Could you check a few things on this model? Use its own coordinates, in mm. A direction names the side the tool comes from. Give positions to 0.01 mm unless a question says otherwise; leave off trailing zeros. Write each loop counter-clockwise with the first axis right and the second up, starting at its lowest first coordinate (ties: lowest second). Pieces come first, ordered by that corner, then holes. Notation, with made-up numbers: M 56,36.25 L 109,36.25 A16 ccw 109,58.25 Z; hole C 11,57.25 d1. An arc over 180 degrees is marked long. Use one line per item in the form item = value.
from build123d import *

# Parameters (mm, degrees)
F0_W          = 250
F0_H          = 52
F1_DEPTH      = 19.2
F2_SIZE2      = 2.017991
F2_SIZE       = 19.19999
F3_SIZE2      = 2.017991
F3_SIZE       = 19.19999
F4_R          = 6.5
F5_DEPTH      = 1.7951503396
F7_DEPTH      = 58.4841370583
F7_DEPTH_BACK = 301.5629071742
F8_R          = 0.55
F9_DEPTH      = 0.5
F10_R         = 0.49999
F11_R         = 0.49999
F12_R         = 13.25
F13_DEPTH     = 4
F14_W         = 21
F14_H         = 8
F14_H_2       = 8.9314985695
F15_DEPTH     = 4


# Not quite as in the source:
# - a fillet or chamfer is up to 0.001 mm smaller than in the source, because OpenCascade refuses the exact size


with BuildPart() as f1:
    # F0 (on Top) → F1 (new body)
    with BuildSketch(Plane.XY):
        with Locations((-1.4450065748, 26)):
            Rectangle(F0_W, F0_H)
    extrude(amount=F1_DEPTH)

    # F2 (size 19.2 and 2.0180013171 in the source; OpenCascade refuses exactly that, so slightly less here)
    f2_edges = [f1.edges().sort_by_distance(p)[0] for p in [
        (-1.445007, 52, 19.2),
    ]]
    f2_side = f1.faces().sort_by_distance((-1.445007, 52, 9.6))[0]
    chamfer(f2_edges, length=F2_SIZE, length2=F2_SIZE2, reference=f2_side)

    # F3 (size 19.2 and 2.0180013171 in the source; OpenCascade refuses exactly that, so slightly less here)
    f3_edges = [f1.edges().sort_by_distance(p)[0] for p in [
        (-1.445007, 0, 19.2),
    ]]
    f3_side = f1.faces().sort_by_distance((-1.445007, 0, 9.6))[0]
    chamfer(f3_edges, length=F3_SIZE, length2=F3_SIZE2, reference=f3_side)

    # F4 (on face) → F5 (cut)
    with BuildSketch(Plane.XY.offset(19.2)):
        with Locations((59.0549934252, 25.9999986829)):
            Circle(F4_R)
    extrude(amount=-F5_DEPTH, mode=Mode.SUBTRACT)

    # F6 (on face) → F7 (cut, two sides)
    with BuildSketch(Plane.YZ.offset(123.5549934252)) as f7_sk:
        Polygon((56.2664195895, -9.8316892982), (52, 0), (0, 0), (-4.1076340713, -9.8316892982), align=None)
        with BuildLine():
            Line((0, 0), (52, 0))
            ThreePointArc((52, 0), (26, 2.5), (0, 0))
        make_face()
    extrude(amount=F7_DEPTH, mode=Mode.SUBTRACT)
    extrude(f7_sk.sketch, amount=-F7_DEPTH_BACK, mode=Mode.SUBTRACT)

    # F8 (on face) → F9 (join)
    with BuildSketch(Plane.XY.offset(19.2)):
        with Locations((120.5049934252, 5.0680013171)):
            Circle(F8_R)
        with Locations((120.5049934252, 46.9319986829)):
            Circle(F8_R)
        with Locations((-120.5049934252, 5.0680013171)):
            Circle(F8_R)
        with Locations((-120.5049934252, 46.9319986829)):
            Circle(F8_R)
    extrude(amount=F9_DEPTH)

    # F10 (radius 0.5 in the source; OpenCascade refuses exactly that, so slightly less here)
    f10_edges = [f1.edges().sort_by_distance(p)[0] for p in [
        (119.954993, 5.068001, 19.7),
    ]]
    fillet(f10_edges, radius=F10_R)

    # F11 (radius 0.5 in the source; OpenCascade refuses exactly that, so slightly less here)
    f11_edges = [f1.edges().sort_by_distance(p)[0] for p in [
        (-121.054993, 5.068001, 19.7),
        (119.954993, 46.931999, 19.7),
        (-121.054993, 46.931999, 19.7),
    ]]
    fillet(f11_edges, radius=F11_R)

    # F12 (on Top) → F13 (cut)
    with BuildSketch(Plane.XY):
        with Locations((-35.1950065748, 26)):
            Circle(F12_R)
    extrude(amount=F13_DEPTH, mode=Mode.SUBTRACT)

    # F14 (on Top) → F15 (cut)
    with BuildSketch(Plane.XY):
        with Locations((48.0549934252, 34.5)):
            Rectangle(F14_W, F14_H)
        with Locations((48.0549934252, 17.9657492848)):
            Rectangle(F14_W, F14_H_2)
    extrude(amount=F15_DEPTH, mode=Mode.SUBTRACT)


solid = f1.part
1) Thinking about a two-plate mould opening in X: for faces 4 (the flat face through (123.555, 26, 9)), 5 (the flat face through (-35, 26, 4)), 6 (the flat face through (48, 18, 4)), 7 (the flat face through (-3.195, 1.023, 9.734)), which applies, released by +X, released by -X, zero draft, split by the parting line, or undercut?
Checked values:
face_4 = released by +X
face_5 = undercut
face_6 = undercut
face_7 = zero draft
2) If I drill on L1, parallel to X at y = 26, z = 2.6 (3 decimals); L2, parallel to X at y = 21.5, z = 3 (3 decimals); L3, parallel to X at y = 20.5, z = 3.25 (3 decimals), over which ranges is the centre line in solid material (lowest first)?
Checked values:
L1 = -126.445 to -48.445, -21.945 to 123.555
L2 = -126.445 to -47.657, -22.733 to 37.555, 58.555 to 123.555
L3 = -126.445 to -47.25, -23.14 to 37.555, 58.555 to 123.555
3) I want a section at B-B, the plane z = 13.5. Please give me the cut outline in (x, y) (3 decimals).
Checked values:
outline = M -126.445,1.419 L 123.555,1.419 L 123.555,50.581 L -126.445,50.581 Z
4) For pin 1 Ø1 at (x, z) = (50, 3) entering from +Y; pin 2 Ø5 at (x, y) = (-70.5, 31) entering from -Z; pin 3 Ø2 at (x, y) = (51.5, 20.5) entering from +Z, each with a flat end and sliding along its axis, tell me the tip position at first contact or that it passes through.
Checked values:
pin_1 = 51.74
pin_2 = 2.29
pin_3 = 19.2
5) I want a section at A-A, the plane x = -102.5. Please give me the cut outline in (y, z), plus the area to 3 significant figures.
Checked values:
outline = M 0,0 A136.45 cw 52,0 L 49.98,19.2 L 2.02,19.2 Z
area = 873 mm2
6) For faces 1 (the cylindrical face through (52.56, 26.29, 18.31)), 2 (the flat face through (48, 35, 4)), 3 (the flat face through (-3.195, 50.977, 9.734)), which set-ups out of +Z, -Z, +X, -X, +Y, -Y let a thin tool reach every point of the face, with its end or its side?
Checked values:
face_1 = +Z
face_2 = -Z
face_3 = +Z, +X, -X, +Y
